Input: part model. Units: mm. Frame: model coordinates. A direction names the side the tool comes from. Give positions to 0.01 mm unless a question says otherwise; leave off trailing zeros. Loops run counter-clockwise (first coordinate to the right, second up) from the corner with the lowest first, then second, coordinate; pieces in that order, holes last. Notation, with made-up numbers: (31.25, 58.5) -> (48.25, 58.5) arc R27 ccw to (48.25, 88.5) -> close; hole circle Ø3 at (35, 42). An arc over 180 degrees is marked (long way). Use CSV: the item, a comma, the result in double quotes.
Autodesk Inventor part; units mm, degrees
ref_plane "YZ Plane" through (0, 0, 0) normal (1, 0, 0) x (0, 1, 0)
ref_plane "XZ Plane" through (0, 0, 0) normal (0, 1, 0) x (-1, 0, 0)
ref_plane "XY Plane" through (0, 0, 0) normal (0, 0, 1) x (1, 0, 0)
sketch "Sketch1" plane through (0, 0, 0) normal (0, 1, 0) x (-1, 0, 0)
  line L0 (95, 271.4286) -> (85, 271.4286)
  line L1 (85, 271.4286) -> (85, -224.5714)
  line L2 (85, -224.5714) -> (95, -224.5714)
  line L3 (95, -224.5714) -> (95, 271.4286)
  point P0 (0, 0)
  dimension "d0" = 10
  dimension "d1" = 496
extrude "Extrusion1" add sketch "Sketch1" along normal blind 250
sketch "Sketch2" plane through (-85, 0, 271.4286) normal (1, 0, 0) x (0, 0, -1)
  line L0 (0, 0) -> (0, 250)
  line L1 (496, 0) -> (496, 250)
  line L2 (0, 218) -> (496, 218)
  line L3 (496, 218) -> (496, 32)
  line L4 (496, 32) -> (0, 32)
  line L5 (0, 32) -> (0, 218)
  line L6 (0, 250) -> (496, 250)
  line L7 (0, 0) -> (496, 0)
  point P0 (271.4286, 0)
  point P1 (0, 32)
  point P2 (496, 218)
  dimension "d4" = 32
  dimension "d5" = 32
  dimension "d6" = 186
extrude "Extrusion3" add sketch "Sketch2" along normal blind 2 contours L0 L4 L1 L7 | L0 L6 L1 L2
sketch "Sketch3" plane through (-95, 0, -224.5714) normal (-1, 0, 0) x (0, 0, 1)
  line L0 (0, 250) -> (496, 250)
  circle A0 centre (248, 250) radius 8
  line L1 (496, 32) -> (496, 218)
  circle A1 centre (496, 125) radius 12
  circle A2 centre (248, 125) radius 32.5
  point P0 (224.5714, 0)
  dimension "d11" = 65
extrude "Extrusion4" cut sketch "Sketch3" against normal blind 35 contours A2
properties part number "Osnova" material "Aluminum 6061"
1) Reachability of faces 5 (the flat face through (-83, 16, 27)), 6 (the flat face through (-85, 82, 27)) from +Z, -Z, +X, -X, +Y, -Y: full face, straight path, thin tool, end or side. Return the list, or none.
From the geometry:
face 5,"+Z, -Z, +X, +Y, -Y"
face 6,"+Z, -Z, +X"
2) Section query C-C (x = -92.75). Return loops of the section in (y, z), then the cut area to 3 significant figures.
From the geometry:
outline,"(0, -224.57) -> (250, -224.57) -> (250, 271.43) -> (0, 271.43) -> close; hole circle Ø65 at (125, 23.43)"
area,"121,000 mm^2"
3) Section query B-B (z = 67). Return loops of the section in (x, y).
From the geometry:
outline,"(-95, 0) -> (-83, 0) -> (-83, 32) -> (-85, 32) -> (-85, 218) -> (-83, 218) -> (-83, 250) -> (-95, 250) -> close"
4) Section query A-A (y = 125). Return loops of the section in (x, z).
From the geometry:
outline,"(-95, -224.57) -> (-85, -224.57) -> (-85, -9.07) -> (-95, -9.07) -> close; (-95, 55.93) -> (-85, 55.93) -> (-85, 271.43) -> (-95, 271.43) -> close"
5) Section query D-D (y = 46.5). Return loops of the section in (x, z), then the cut area to 3 significant figures.
From the geometry:
outline,"(-95, -224.57) -> (-85, -224.57) -> (-85, 271.43) -> (-95, 271.43) -> close"
area,"4,960 mm^2"
6) Ray query, line 1 (Y direction, x = -84, z = 247); line 2 (X direction, y = 213, z = -70); line 3 (Z direction, x = -87, y = 136). Return the intervals inside material, ascending.
From the geometry:
line 1,"y = 0 to 32, 218 to 250"
line 2,"x = -95 to -85"
line 3,"z = -224.57 to -7.15, 54.01 to 271.43"
7) Mould query, pull axis Y, two halves, no side actions, for faces 1 (the flat face through (-89, 0, 27)), 2 (the flat face through (-89, 250, 27)), 3 (the cylindrical face through (-90.07, 93.273, 16.383)), 4 (the flat face through (-90, 123, -224.571)). Classes: pulls with the +Y half, pulls with the -Y half, needs draft (parallel to the pull), parting line crosses it, or undercut.
From the geometry:
face 1,"pulls with the -Y half"
face 2,"pulls with the +Y half"
face 3,"undercut"
face 4,"needs draft"
8) Contact query for a flat-ended pin moving along its axis: pin 1 (4 mm diameter, centred on y = 126, z = -52.5, fed in from +X). Output: stop coordinate, or through.
From the geometry:
pin 1,"stops at x = -85"
